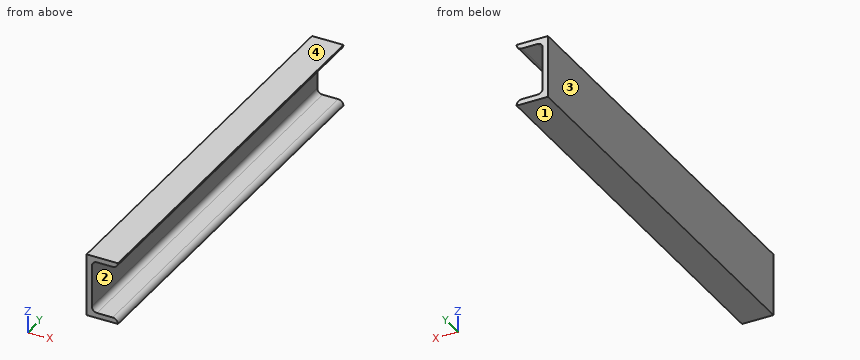
from build123d import *

# Parameters (mm, degrees)
F1_DEPTH = 505.46


# Not quite as in the source:
# - ends of sketch curves that miss each other by under 0.0002 mm in the source are joined


with BuildPart() as f1:
    # F0 (on Front) → F1 (new body)
    with BuildSketch(Plane.XZ):
        with BuildLine():
            Line((0, 76.2), (0, 0))
            Line((0, 0), (38.1, 0))
            ThreePointArc((38.1, 0), (36.2401280605, 4.4901312434), (31.75, 6.3500031829))
            Line((31.75, 6.3500031829), (12.7000031829, 6.3500031829))
            ThreePointArc((12.7000031829, 6.3500031829), (8.2098751224, 8.2098751224), (6.3500031829, 12.7000031829))
            Line((6.3500031829, 12.7000031829), (6.3500031829, 63.4999968171))
            ThreePointArc((6.3500031829, 63.4999968171), (8.2098751224, 67.9901248776), (12.7000031829, 69.8499968171))
            Line((12.7000031829, 69.8499968171), (31.75, 69.8499968171))
            ThreePointArc((31.75, 69.8499968171), (36.2401280605, 71.7098687566), (38.1, 76.1999968171))
            Line((38.1, 76.1999968171), (0, 76.2))
        make_face()
    extrude(amount=F1_DEPTH)


solid = f1.part
Check sheet for the modelled part. Datum: model origin and axes. Units: mm. Face numbers are marked on the shaded views. Round coordinates to 2 decimals unless told otherwise and drop trailing zeros. Order: outer loops, then holes, each group sorted by start corner. A loop starts at its lowest first (then second) coordinate and runs counter-clockwise, first axis right, second up.
(1) Draft check along Z on the marked faces 1, 2, 3 and 4. Enter one of: pulls with the +Z half, pulls with the -Z half, needs draft (parallel to the pull), parting line crosses it, or undercut.
(2) Cross-section at B-B, the plane y = -320. Enter the section's corners in (x, z), and give its area (3 significant figures).
(3) Cross-section at C-C, the plane z = 17. Enter the section's corners in (x, y).
(4) Go/stop test with flat-tipped pins: P1, Ø1, axis at y = -65, z = 18.5, coming from the +X side; P2, Ø6, axis at x = 15.5, z = 64.5, coming from the +Y side. Record where each tip stops, or that it passes through.
(5) Cross-section at A-A, the plane x = 22. Enter the section's corners in (y, z).
(6) Scan lines: probe 1 along Z at (x, y) = (32.5, -465); probe 2 along Z at (x, y) = (28, -115); probe 3 along X at (y, z) = (-145.5, 21). Record each from-to range of solid material in increasing order.
Check sheet entries:
1. face 1: pulls with the -Z half
1. face 2: undercut
1. face 3: needs draft
1. face 4: pulls with the +Z half
2. outline: (0, 0) - (38.1, 0) arc R6.35 ccw to (31.75, 6.35) - (12.7, 6.35) arc R6.35 cw to (6.35, 12.7) - (6.35, 63.5) arc R6.35 cw to (12.7, 69.85) - (31.75, 69.85) arc R6.35 ccw to (38.1, 76.2) - (0, 76.2) - close
2. area: 887 mm2
3. outline: (0, -505.46) - (6.35, -505.46) - (6.35, 0) - (0, 0) - close
4. P1: stops at x = 6.35
4. P2: passes through
5. outline: (-505.46, 0) - (0, 0) - (0, 6.35) - (-505.46, 6.35) - close; (-505.46, 69.85) - (0, 69.85) - (0, 76.2) - (-505.46, 76.2) - close
6. probe 1: z = 0 to 6.31, 69.89 to 76.2
6. probe 2: z = 0 to 6.35, 69.85 to 76.2
6. probe 3: x = 0 to 6.35
